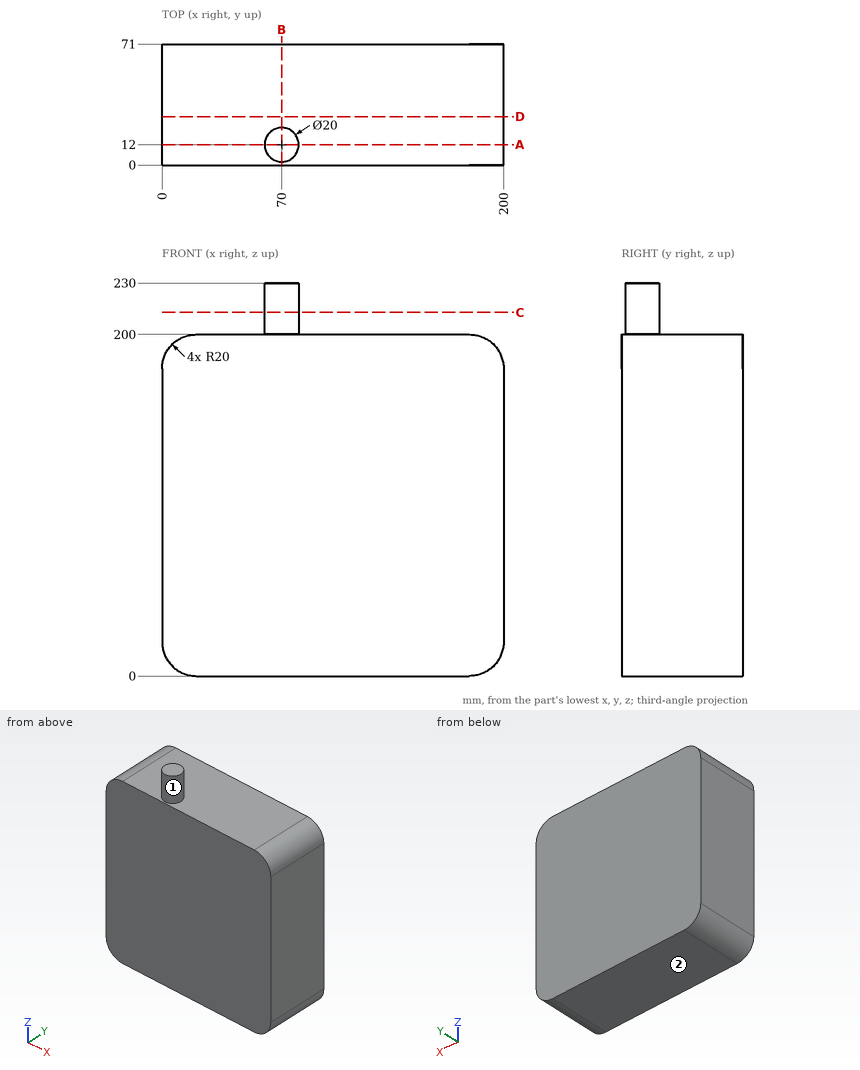
Verification items for this drawing (mm, ordinates from the low corner). A direction names the side the tool comes from. Round coordinates to 2 decimals unless told otherwise and drop trailing zeros. Order: outer loops, then holes, each group sorted by start corner. A loop starts at its lowest first (then second) coordinate and runs counter-clockwise, first axis right, second up. Notation, with made-up numbers: (53, 39.5) - (108, 39.5) arc R17 cw to (108, 60.5) - close; hole circle Ø1 at (32.5, -3.5). An arc over 180 degrees is marked (long way). Answer as CSV lines item,"result". Start each with the question number.
1) Section check C-C (z = 213). Record the cut outline in (x, y), then the cut area to 3 significant figures.
2) Depth check by flat-ended pin: pin 1 (12 mm diameter, centred on x = 165.5, y = 42, fed in from +Z). Enter the tip coordinate at first touch or a pass-through.
3) Tool access check on the marked faces 1 and 2. Record the directions out of +Z, -Z, +X, -X, +Y, -Y that give a thin tool (end or side, any length) a straight path to the whole face; none if there is none.
4) Section check A-A (y = 12). Record the cut outline in (x, z), then the cut area to 3 significant figures.
5) Scan lines: probe 1 along Z at (x, y) = (164.5, 15.5); probe 2 along Z at (x, y) = (187.5, 49); probe 3 along X at (y, z) = (66, 198.5). Record each from-to range of solid material in increasing order.
6) Section check D-D (y = 28.5). Record the cut outline in (x, z), then the cut area to 3 significant figures.
7) Section check B-B (x = 70). Record the cut outline in (y, z).
Determined:
1,outline,"circle Ø20 at (70, 12)"
1,area,"314 mm^2"
2,pin 1,"z = 200"
3,face 1,"+Z"
3,face 2,"-Z, +X, -X, +Y, -Y"
4,outline,"(0, 20) arc R20 ccw to (20, 0) - (180, 0) arc R20 ccw to (200, 20) - (200, 180) arc R20 ccw to (180, 200) - (80, 200) - (80, 230) - (60, 230) - (60, 200) - (20, 200) arc R20 ccw to (0, 180) - close"
4,area,"40,300 mm^2"
5,probe 1,"0 to 200"
5,probe 2,"1.46 to 198.54"
5,probe 3,"12.4 to 187.6"
6,outline,"(0, 20) arc R20 ccw to (20, 0) - (180, 0) arc R20 ccw to (200, 20) - (200, 180) arc R20 ccw to (180, 200) - (20, 200) arc R20 ccw to (0, 180) - close"
6,area,"39,700 mm^2"
7,outline,"(0, 0) - (71, 0) - (71, 200) - (22, 200) - (22, 230) - (2, 230) - (2, 200) - (0, 200) - close"
